Design review of the part built by this model. Coordinates are the model's own, in mm. A direction names the side the tool comes from. Coordinates: 2 decimals unless noted, no trailing zeros. Loops run counter-clockwise (first coordinate to the right, second up) from the corner with the lowest first, then second, coordinate; pieces in that order, holes last.
Q1. Machinability: for faces 5 (the face through (1, 3, 225.548)), 6 (the face through (97.37, 3.131, 95.127)), 7 (the face through (-20.479, 3, 201)), which of the approach directions +Z, -Z, +X, -X, +Y, -Y give a long, thin tool a straight path to every point of the face, cutting with its end or side? Answer none if there is none.
Q2. Add section B-B on x = -40.5. Give the boundary of the cut face in (y, z).
Q3. Draft analysis for pull direction Z (two halves, no side actions). For faces 1 (the face through (128.71, 3.13, 131.7)), 2 (the face through (30, 3, 150.474)), 3 (the face through (-30, 3, 131.424)), 4 (the face through (67.02, 3.22, 157.81)), state which applies: released by +Z, released by -Z, zero draft, split by the parting line, or undercut.
Q4. Add section C-C on y = 4. Give the number of separate pieces and of enclosed holes in the cut face, and give its area (3 significant figures).
Q5. For P1, Ø2.5, axis at x = -33.18, z = 158.75, coming from the -Y side; P2, Ø2, axis at x = -74, y = 4.5, coming from the -Z side; P3, Ø1, axis at x = 79.5, y = 2, coming from the -Z side; P4, Ø3, axis at x = 29, y = 2.5, coming from the -Z side, all flat-tipped, find the tip position at first contact; note any pin that passes through.
Q6. Add section A-A on x = 117.5. Give the boundary of the cut face in (y, z), and give its area (3 significant figures).
Q7. Wall thickness on probe 1 along Z at (x, y) = (-29.5, 4.25); probe 2 along X at (y, z) = (2.75, 155); probe 3 along X at (y, z) = (6, 123.5): over which ranges is each line inside the solid? List them lowest first.
```python
from build123d import *

# Parameters (mm, degrees)
BOSS_EXTRUDE1_DEPTH    = 6.35
FILLET4_R              = 3.175
F_10_CLEARANCE_HOLE1_D = 5.1054
CUT_EXTRUDE1_DEPTH     = 278.292988553
FILLET5_R              = 12.7
SKETCH5_R              = 1.5875
CUT_EXTRUDE2_DEPTH     = 278.292988553
CUT_EXTRUDE3_DEPTH     = 278.292988553


with BuildPart() as part:
    # Sketch1 → Boss-Extrude1 (new body)
    with BuildSketch(Plane(origin=(0, 0, 0), x_dir=(1, 0, 0), z_dir=(0, 1, 0))):
        with BuildLine():
            Line((33.17875, -158.75), (33.17875, -153.648789236))
            ThreePointArc((33.17875, -153.648789236), (34.76625, -152.061289236), (33.17875, -150.473789236))
            Line((33.17875, -150.473789236), (26.82875, -150.473789236))
            Line((26.82875, -150.473789236), (26.82875, -131.423789236))
            Line((26.82875, -131.423789236), (33.17875, -131.423789236))
            ThreePointArc((33.17875, -131.423789236), (34.76625, -129.836289236), (33.17875, -128.248789236))
            Line((33.17875, -128.248789236), (33.17875, -122.589438976))
            ThreePointArc((33.17875, -122.589438976), (43.137840894, -119.449264054), (52.805287488, -115.501522126))
            Line((52.805287488, -115.501522126), (143.19952673, -74.174847787))
            ThreePointArc((143.19952673, -74.174847787), (157.875678173, -77.180277992), (159.478578107, -92.075))
            ThreePointArc((159.478578107, -92.075), (128.201088688, -132.195700986), (87.13986874, -162.227820598))
            ThreePointArc((87.13986874, -162.227820598), (59.463291006, -188.659212722), (49.275, -225.54837334))
            Line((49.275, -225.54837334), (-49.275, -225.54837334))
            ThreePointArc((-49.275, -225.54837334), (-59.463291006, -188.659212722), (-87.13986874, -162.227820598))
            ThreePointArc((-87.13986874, -162.227820598), (-128.201088688, -132.195700986), (-159.478578107, -92.075))
            ThreePointArc((-159.478578107, -92.075), (-157.875678173, -77.180277992), (-143.19952673, -74.174847787))
            Line((-143.19952673, -74.174847787), (-52.805287488, -115.501522126))
            ThreePointArc((-52.805287488, -115.501522126), (-43.137840894, -119.449264054), (-33.17875, -122.589438976))
            Line((-33.17875, -122.589438976), (-33.17875, -128.248789236))
            ThreePointArc((-33.17875, -128.248789236), (-34.76625, -129.836289236), (-33.17875, -131.423789236))
            Line((-33.17875, -131.423789236), (-26.82875, -131.423789236))
            Line((-26.82875, -131.423789236), (-26.82875, -150.473789236))
            Line((-26.82875, -150.473789236), (-33.17875, -150.473789236))
            ThreePointArc((-33.17875, -150.473789236), (-34.76625, -152.061289236), (-33.17875, -153.648789236))
            Line((-33.17875, -153.648789236), (-33.17875, -158.75))
            Line((-33.17875, -158.75), (33.17875, -158.75))
        make_face()
    extrude(amount=BOSS_EXTRUDE1_DEPTH)

    # Fillet4
    fillet4_edges = [part.edges().sort_by_distance(p)[0] for p in [
        (33.17875, 3.175, 122.589438976),
        (-33.17875, 3.175, 122.589438976),
    ]]
    fillet(fillet4_edges, radius=FILLET4_R)

    # #10 Clearance Hole1 (through all)
    with Locations(Plane(origin=(0, 6.35, 0), x_dir=(1, 0, 0), z_dir=(0, 1, 0))):
        with Locations((-151.12143296, -87.25), (-87.25, -151.12143296), (87.25, -151.12143296), (151.12143296, -87.25), (0, -174.5)):
            Hole(F_10_CLEARANCE_HOLE1_D / 2)

    # Sketch4 → Cut-Extrude1 (cut, through all)
    with BuildSketch(Plane(origin=(0, 6.35, 0), x_dir=(1, 0, 0), z_dir=(0, 1, 0))):
        with BuildLine():
            Line((-23.754817001, -214.08399668), (-29.902682999, -214.08399668))
            ThreePointArc((-29.902682999, -214.08399668), (-31.540716499, -215.722030181), (-33.17875, -214.08399668))
            Line((-33.17875, -214.08399668), (-33.17875, -188.68399668))
            ThreePointArc((-33.17875, -188.68399668), (-31.540716499, -187.045963179), (-29.902682999, -188.68399668))
            Line((-29.902682999, -188.68399668), (-23.754817001, -188.68399668))
            ThreePointArc((-23.754817001, -188.68399668), (-22.116783501, -187.045963179), (-20.47875, -188.68399668))
            Line((-20.47875, -188.68399668), (-20.47875, -214.08399668))
            ThreePointArc((-20.47875, -214.08399668), (-22.116783501, -215.722030181), (-23.754817001, -214.08399668))
        make_face()
        with BuildLine():
            Line((23.754817001, -214.08399668), (29.902682999, -214.08399668))
            ThreePointArc((29.902682999, -214.08399668), (31.540716499, -215.722030181), (33.17875, -214.08399668))
            Line((33.17875, -214.08399668), (33.17875, -188.68399668))
            ThreePointArc((33.17875, -188.68399668), (31.540716499, -187.045963179), (29.902682999, -188.68399668))
            Line((29.902682999, -188.68399668), (23.754817001, -188.68399668))
            ThreePointArc((23.754817001, -188.68399668), (22.116783501, -187.045963179), (20.47875, -188.68399668))
            Line((20.47875, -188.68399668), (20.47875, -214.08399668))
            ThreePointArc((20.47875, -214.08399668), (22.116783501, -215.722030181), (23.754817001, -214.08399668))
        make_face()
    extrude(amount=-CUT_EXTRUDE1_DEPTH, mode=Mode.SUBTRACT)

    # Fillet5
    fillet5_edges = [part.edges().sort_by_distance(p)[0] for p in [
        (-49.275, 3.175, 225.54837334),
        (49.275, 3.175, 225.54837334),
    ]]
    fillet(fillet5_edges, radius=FILLET5_R)

    # Sketch5 → Cut-Extrude2 (cut, through all)
    with BuildSketch(Plane(origin=(0, 6.35, 0), x_dir=(1, 0, 0), z_dir=(0, 1, 0))):
        with Locations((33.17875, -158.75)):
            Circle(SKETCH5_R)
        with Locations((-33.17875, -158.75)):
            Circle(SKETCH5_R)
    extrude(amount=-CUT_EXTRUDE2_DEPTH, mode=Mode.SUBTRACT)

    # Sketch6 → Cut-Extrude3 (cut, through all)
    with BuildSketch(Plane(origin=(0, 6.35, 0), x_dir=(1, 0, 0), z_dir=(0, 1, 0))):
        with BuildLine():
            Line((-128.104892872, -95.040170045), (-102.637452085, -106.683441126))
            ThreePointArc((-102.637452085, -106.683441126), (-97.569832685, -110.871132479), (-95.274991225, -117.031589274))
            Line((-95.274991225, -117.031589274), (-93.991682853, -130.529758616))
            ThreePointArc((-93.991682853, -130.529758616), (-97.23388696, -136.684180208), (-104.171376798, -136.174251443))
            ThreePointArc((-104.171376798, -136.174251443), (-121.000806478, -121.465663179), (-135.773817141, -104.692755619))
            ThreePointArc((-135.773817141, -104.692755619), (-135.716998993, -96.865146197), (-128.104892872, -95.040170045))
        make_face()
        with BuildLine():
            Line((75.963518128, -118.878299904), (53.298221251, -129.240479515))
            ThreePointArc((53.298221251, -129.240479515), (47.89341624, -133.926693904), (45.87875, -140.790631728))
            Line((45.87875, -140.790631728), (45.87875, -147.546916431))
            ThreePointArc((45.87875, -147.546916431), (51.445237892, -158.054199858), (63.26505, -159.350669746))
            ThreePointArc((63.26505, -159.350669746), (67.071533898, -157.786285337), (70.839373095, -156.130988979))
            ThreePointArc((70.839373095, -156.130988979), (73.48252349, -153.895611155), (74.56046174, -150.606050825))
            ThreePointArc((74.56046174, -150.606050825), (75.950573651, -145.323764103), (79.430821218, -141.113913629))
            ThreePointArc((79.430821218, -141.113913629), (82.749836121, -137.208085982), (84.254632043, -132.308398362))
            Line((84.254632043, -132.308398362), (84.925277307, -125.254378043))
            ThreePointArc((84.925277307, -125.254378043), (82.285012932, -119.479301937), (75.963518128, -118.878299904))
        make_face()
        with BuildLine():
            Line((93.991682853, -130.529758616), (95.274991225, -117.031589274))
            ThreePointArc((95.274991225, -117.031589274), (97.569832685, -110.871132479), (102.637452085, -106.683441126))
            Line((102.637452085, -106.683441126), (128.104892872, -95.040170045))
            ThreePointArc((128.104892872, -95.040170045), (135.716998993, -96.865146197), (135.773817141, -104.692755619))
            ThreePointArc((135.773817141, -104.692755619), (121.000806478, -121.465663179), (104.171376798, -136.174251443))
            ThreePointArc((104.171376798, -136.174251443), (97.23388696, -136.684180208), (93.991682853, -130.529758616))
        make_face()
        with BuildLine():
            Line((-45.87875, -140.790631728), (-45.87875, -147.546916431))
            ThreePointArc((-45.87875, -147.546916431), (-51.445237892, -158.054199858), (-63.26505, -159.350669746))
            ThreePointArc((-63.26505, -159.350669746), (-67.071533898, -157.786285337), (-70.839373095, -156.130988979))
            ThreePointArc((-70.839373095, -156.130988979), (-73.48252349, -153.895611155), (-74.56046174, -150.606050825))
            ThreePointArc((-74.56046174, -150.606050825), (-75.950573651, -145.323764103), (-79.430821218, -141.113913629))
            ThreePointArc((-79.430821218, -141.113913629), (-82.749836121, -137.208085982), (-84.254632043, -132.308398362))
            Line((-84.254632043, -132.308398362), (-84.925277307, -125.254378043))
            ThreePointArc((-84.925277307, -125.254378043), (-82.285012932, -119.479301937), (-75.963518128, -118.878299904))
            Line((-75.963518128, -118.878299904), (-53.298221251, -129.240479515))
            ThreePointArc((-53.298221251, -129.240479515), (-47.89341624, -133.926693904), (-45.87875, -140.790631728))
        make_face()
    extrude(amount=-CUT_EXTRUDE3_DEPTH, mode=Mode.SUBTRACT)


solid = part.part
```
Entries:
1. face 5: +Z, +X, -X, +Y, -Y
1. face 6: -Z, +Y, -Y
1. face 7: +Y, -Y
2. outline: (0, 120.37) - (6.35, 120.37) - (6.35, 225.2) - (0, 225.2) - close
3. face 1: released by +Z
3. face 2: undercut
3. face 3: released by -Z
3. face 4: undercut
4. separate pieces: 1
4. enclosed holes: 11
4. area: 15,700 mm2
5. P1: passes through
5. P2: stops at z = 105.35
5. P3: stops at z = 103.07
5. P4: stops at z = 131.42
6. outline: (0, 85.92) - (6.35, 85.92) - (6.35, 99.89) - (0, 99.89) - close; (0, 124.86) - (6.35, 124.86) - (6.35, 141.79) - (0, 141.79) - close
6. area: 196 mm2
7. probe 1: z = 131.42 to 150.47, 158.75 to 188.68, 214.08 to 225.55
7. probe 2: x = -99.43 to -72.54, -48.3 to -33.18, 33.18 to 48.3, 72.54 to 99.43
7. probe 3: x = -136.6 to -118.92, -94.66 to -84.85, -65.85 to -33.55, 33.55 to 65.85, 84.85 to 94.66, 118.92 to 136.6
